from build123d import *

# Parameters (mm, degrees)
SKETCH1_W           = 20
SKETCH1_H           = 20
BOSS_EXTRUDE1_DEPTH = 5
CUT_EXTRUDE1_REACH  = 24.913
SKETCH2_R           = 3.1
CUT_EXTRUDE2_REACH  = 17
SKETCH3_R           = 2


with BuildPart() as part:
    # Sketch1 → Boss-Extrude1 (new body)
    with BuildSketch(Plane.XY):
        Rectangle(SKETCH1_W, SKETCH1_H)
    extrude(amount=BOSS_EXTRUDE1_DEPTH)

    # Sketch2 → Cut-Extrude1 (cut, up to next)
    with BuildSketch(Plane(origin=(0, 10, 0), x_dir=(1, 0, 0), z_dir=(0, 1, 0)), mode=Mode.PRIVATE) as cut_extrude1_sk1:
        Circle(SKETCH2_R)
    cut_extrude1_tool1 = extrude(cut_extrude1_sk1.sketch, amount=-CUT_EXTRUDE1_REACH, mode=Mode.PRIVATE) & part.part
    add(cut_extrude1_tool1.solids().sort_by_distance((0, 10, 0))[0], mode=Mode.SUBTRACT)

    # Sketch3 → Cut-Extrude2 (cut, up to next)
    with BuildSketch(Plane.XY.offset(5), mode=Mode.PRIVATE) as cut_extrude2_sk1:
        with Locations((-6, 6)):
            Circle(SKETCH3_R)
    cut_extrude2_tool1 = extrude(cut_extrude2_sk1.sketch, amount=-CUT_EXTRUDE2_REACH, mode=Mode.PRIVATE) & part.part
    # Sketch3 → Cut-Extrude2 (cut, up to next)
    with BuildSketch(Plane.XY.offset(5), mode=Mode.PRIVATE) as cut_extrude2_sk2:
        with Locations((-6, -6)):
            Circle(SKETCH3_R)
    cut_extrude2_tool2 = extrude(cut_extrude2_sk2.sketch, amount=-CUT_EXTRUDE2_REACH, mode=Mode.PRIVATE) & part.part
    # Sketch3 → Cut-Extrude2 (cut, up to next)
    with BuildSketch(Plane.XY.offset(5), mode=Mode.PRIVATE) as cut_extrude2_sk3:
        with Locations((6, -6)):
            Circle(SKETCH3_R)
    cut_extrude2_tool3 = extrude(cut_extrude2_sk3.sketch, amount=-CUT_EXTRUDE2_REACH, mode=Mode.PRIVATE) & part.part
    # Sketch3 → Cut-Extrude2 (cut, up to next)
    with BuildSketch(Plane.XY.offset(5), mode=Mode.PRIVATE) as cut_extrude2_sk4:
        with Locations((6, 6)):
            Circle(SKETCH3_R)
    cut_extrude2_tool4 = extrude(cut_extrude2_sk4.sketch, amount=-CUT_EXTRUDE2_REACH, mode=Mode.PRIVATE) & part.part
    add(cut_extrude2_tool1.solids().sort_by_distance((-6, 6, 5))[0], mode=Mode.SUBTRACT)
    add(cut_extrude2_tool2.solids().sort_by_distance((-6, -6, 5))[0], mode=Mode.SUBTRACT)
    add(cut_extrude2_tool3.solids().sort_by_distance((6, -6, 5))[0], mode=Mode.SUBTRACT)
    add(cut_extrude2_tool4.solids().sort_by_distance((6, 6, 5))[0], mode=Mode.SUBTRACT)


solid = part.part
Design review of the part built by this model. Coordinates are the model's own, in mm. Give positions to 0.01 mm unless a question says otherwise; leave off trailing zeros. Order: outer loops, then holes, each group sorted by start corner. A loop starts at its lowest first (then second) coordinate and runs counter-clockwise, first axis right, second up. Notation, with made-up numbers: (-5.75, -26.5) - (6.25, -26.5) arc R33 ccw to (6.25, 9.5) - close; hole circle Ø4 at (-35, 82.5). An arc over 180 degrees is marked (long way). Use CSV: the item, a comma, the result in double quotes. Start each with the question number.
Q1. Take a section at D-D (y = -2.25). State the section outline as (x, z) points.
Q2. Take a section at A-A (x = 6). State the section outline as (y, z) points.
Q3. Draft analysis for pull direction X (two halves, no side actions). For faces 1 (the face through (10, 0, 2)), 2 (the face through (4.4, -7.2, 2.5)), 3 (the face through (-7, 0, 0)), state which applies: pulls with the +X half, pulls with the -X half, needs draft (parallel to the pull), parting line crosses it, or undercut.
Q4. For line 1 (Y direction, x = 6, z = 1.5); line 2 (X direction, y = 6.5, z = 4.1); line 3 (Y direction, x = -7.5, z = 4.1), list the stretches that pass through material, from the lowest coordinate up.
Q5. Take a section at B-B (y = -6). State the section outline as (x, z) points.
Q6. Take a section at C-C (z = 1.35). State the section outline as (x, y) points.
Calculated:
1,outline,"(-10, 0) - (-3.1, 0) arc R3.1 cw to (3.1, 0) - (10, 0) - (10, 5) - (-10, 5) - close"
2,outline,"(-10, 0) - (-8, 0) - (-8, 5) - (-10, 5) - close; (-4, 0) - (4, 0) - (4, 5) - (-4, 5) - close; (8, 0) - (10, 0) - (10, 5) - (8, 5) - close"
3,face 1,"pulls with the +X half"
3,face 2,"undercut"
3,face 3,"needs draft"
4,line 1,"y = -10 to -8, -4 to 4, 8 to 10"
4,line 2,"x = -10 to -7.94, -4.06 to 4.06, 7.94 to 10"
4,line 3,"y = -10 to -7.32, -4.68 to 4.68, 7.32 to 10"
5,outline,"(-10, 0) - (-8, 0) - (-8, 5) - (-10, 5) - close; (-4, 0) - (-3.1, 0) arc R3.1 cw to (3.1, 0) - (4, 0) - (4, 5) - (-4, 5) - close; (8, 0) - (10, 0) - (10, 5) - (8, 5) - close"
6,outline,"(-10, -10) - (-2.79, -10) - (-2.79, 10) - (-10, 10) - close; (2.79, -10) - (10, -10) - (10, 10) - (2.79, 10) - close; hole circle Ø4 at (-6, -6); hole circle Ø4 at (-6, 6); hole circle Ø4 at (6, -6); hole circle Ø4 at (6, 6)"
